Autodesk Inventor part; units mm, degrees
ref_plane "YZ Plane" through (0, 0, 0) normal (1, 0, 0) x (0, 1, 0)
ref_plane "XZ Plane" through (0, 0, 0) normal (0, 1, 0) x (-1, 0, 0)
ref_plane "XY Plane" through (0, 0, 0) normal (0, 0, 1) x (1, 0, 0)
sketch "Sketch1" plane through (0, 0, 0) normal (0, 0, 1) x (1, 0, 0)
  line L0 (2, 0) -> (65, 0)
  line L1 (65, 0) -> (65, 29)
  line L2 (65, 29) -> (2, 29)
  line L3 (0, 27) -> (0, 2)
  arc A0 (2, 29) -> (0, 27) centre (2, 27) ccw
  arc A1 (0, 2) -> (2, 0) centre (2, 2) ccw
  line L4 (20, 29) -> (20, 0)
  line L5 (55, 29) -> (55, 0)
  circle A2 centre (7, 24.5) radius 1.5
  circle A3 centre (7, 4.5) radius 1.5
  circle A4 centre (13.5, 24.5) radius 1.5
  circle A5 centre (13.5, 4.5) radius 1.5
  line L6 (65, 0) -> (65, -2.5)
  line L7 (65, -2.5) -> (55, -2.5)
  line L8 (55, -2.5) -> (55, 0)
  line L9 (55, 29) -> (55, 31.5)
  line L10 (55, 31.5) -> (65, 31.5)
  line L11 (65, 31.5) -> (65, 29)
  point P0 (0, 0)
  point P1 (0, 29)
  dimension "d0" = 65
  dimension "d1" = 29
  dimension "d2" = 2
  dimension "d3" = 20
  dimension "d4" = 10
  dimension "d5" = 3
  dimension "d6" = 3
  dimension "d7" = 4.5
  dimension "d8" = 4.5
  dimension "d9" = 20
  dimension "d10" = 3
  dimension "d11" = 3
  dimension "d12" = 20
  dimension "d13" = 6.5
  dimension "d14" = 7
  dimension "d24" = 2.5
  dimension "d25" = 2.5
extrude "Extrusion1" add sketch "Sketch1" along normal blind 5 contours L4 L2 L5 L0
extrude "Extrusion2" add sketch "Sketch1" along normal blind 7 contours A1 L3 A0 L2 L4 L0
extrude "Extrusion3" add sketch "Sketch1" along normal blind 26.25 contours L5 L2 L1 L0
sketch "Sketch2" plane through (55, 0, 5) normal (-1, 0, 0) x (0, 0, 1)
  line L0 (21.25, 29) -> (21.25, 0)
  circle A0 centre (21.25, 14.5) radius 10
  point P0 (-5, 0)
  point P1 (21.25, 4.5)
  point P2 (21.25, 24.5)
  dimension "d21" = 20
extrude "Extrusion4" cut sketch "Sketch2" against normal blind 20 contours L0 A0 picked at (15.0351, 13.318)
extrude "Extrusion5" add sketch "Sketch1" along normal blind 26.25 contours L0 L6 L7 L8 | L9 L10 L11 L2
sketch "Sketch4" plane through (55, 0, 5) normal (-1, 0, 0) x (0, 0, 1)
  circle A0 centre (13.75, 1.5095) radius 2.05
  circle A1 centre (13.75, 27.4905) radius 2.05
  line L0 (-5, -2.5) -> (21.25, -2.5)
  line L1 (-5, 31.5) -> (21.25, 31.5)
  line L2 (21.25, 31.5) -> (21.25, 24.5)
  point P0 (-5, 0)
  point P1 (8.125, -2.5)
  dimension "d28" = 4.1
  dimension "d29" = 4.1
  dimension "d30" = 25.981
  dimension "d31" = 4.0095
  dimension "d32" = 4.0095
  dimension "d33" = 7.5
extrude "Extrusion6" cut sketch "Sketch4" against normal blind 26.25
chamfer "Chamfer1" distance 2.5 angle 45 1 edges at (55, 0, 2.5)
chamfer "Chamfer2" distance 2.5 angle 45 1 edges at (55, 29, 2.5)
chamfer "Chamfer3" distance 6 angle 45 1 edges at (55, 14.5, 5)
chamfer "Chamfer4" distance 0.6 angle 45 6 edges at (20, 14.5, 7) (11, 0, 7) (0.5858, 0.5858, 7) (0, 14.5, 7) (0.5858, 28.4142, 7) (11, 29, 7)
equation "\"BendRadius\" = Thickness"
equation "\"BendReliefWidth\" = Thickness"
equation "\"BendReliefDepth\" = 0.5 * Thickness"
equation "\"CornerReliefSize\" = 4 * Thickness"
equation "\"MinimumRemnant\" = 2 * Thickness"
equation "\"TransitionRadius\" = BendRadius"
equation "\"JacobiRadiusSize\" = BendRadius"
equation "\"GapSize\" = Thickness"
properties part number "tool4_1"
The listing builds one solid part. Answer for the finished solid, in the listing's coordinates (mm). A direction names the side the tool comes from. Give positions to 0.01 mm unless a question says otherwise; leave off trailing zeros. Order: outer loops, then holes, each group sorted by start corner. A loop starts at its lowest first (then second) coordinate and runs counter-clockwise, first axis right, second up. Notation, with made-up numbers: (-36.75, 22) -> (-7.75, 22) arc R7 ccw to (-7.75, 26) -> close; hole circle Ø4 at (-17, 54.25). An arc over 180 degrees is marked (long way). Answer as a JSON object with one key per item and string values. Group by question number.
Item 1: A tool of negligible diameter and unlimited length cuts with its end or side. For faces 5 (the flat face through (10, 15, 7)), 6 (the cylindrical face through (12.39, 23.49, 3.45)), 7 (the flat face through (52, 14, 8)), from which of +Z, -Z, +X, -X, +Y, -Y can it reach the whole face along a straight path? Write none if from no direction.
Item 2: The part is cut by section B-B on z = 20. Write down the section's boundary in (x, y).
Item 3: Flat-ended cylindrical pins translate along their axes: pin 1 (6.5 mm diameter, centred on y = 1.51, z = 18.75, fed in from -X); pin 2 (5 mm diameter, centred on x = 13.5, y = 24.5, fed in from +Z); pin 3 (12 mm diameter, centred on x = 43.5, z = 5, fed in from -Y). Find the tip coordinate at first contact, or state that the pin passes through.
Item 4: The part is cut by section D-D on y = 14.5. Write down the section's boundary in (x, z), and give its area (3 significant figures).
Item 5: The part is cut by section A-A on x = 13.5. Write down the section's boundary in (y, z).
Item 6: Consider L1, parallel to Y at x = 7, z = 5.25; L2, parallel to X at y = 24, z = 3; L3, parallel to Y at x = 58.75, z = 18.75. Determine where each line is inside the solid, lowest interval first. Write a range as from..to.
Item 7: The part is cut by section C-C on z = 24.5. Write down the section's boundary in (x, y), and give its area (3 significant figures).
Item 8: Determine the mould class of faces 1 (the flat face through (34, 15, 5)), 2 (the flat face through (28, 29, 2)), 3 (the flat face through (53.7, 30.2, 5.4)), 4 (the flat face through (20, 15, 6)) for opening direction X: pulls with the +X half, pulls with the -X half, needs draft (parallel to the pull), parting line crosses it, or undercut.
Result set:
{
 "1": {"face 5": "+Z, -X, +Y, -Y", "face 6": "+Z, -Z", "face 7": "+Z, +Y, -Y"},
 "2": {"outline": "(55, -2.5) -> (65, -2.5) -> (65, -0.12) -> (55, -0.12) -> close; (55, 3.13) -> (65, 3.13) -> (65, 6.69) -> (55, 6.69) -> close; (55, 22.31) -> (65, 22.31) -> (65, 25.87) -> (55, 25.87) -> close; (55, 29.12) -> (65, 29.12) -> (65, 31.5) -> (55, 31.5) -> close"},
 "3": {"pin 1": "x = 55", "pin 2": "z = 7", "pin 3": "y = 0"},
 "4": {"outline": "(0, 0) -> (65, 0) -> (65, 16.25) -> (55, 16.25) -> (55, 11) -> (49, 5) -> (20, 5) -> (20, 6.4) -> (19.4, 7) -> (0.6, 7) -> (0, 6.4) -> close", "area": "495 mm²"},
 "5": {"outline": "(0, 0) -> (3, 0) -> (3, 7) -> (0.6, 7) -> (0, 6.4) -> close; (6, 0) -> (23, 0) -> (23, 7) -> (6, 7) -> close; (26, 0) -> (29, 0) -> (29, 6.4) -> (28.4, 7) -> (26, 7) -> close"},
 "6": {"L1": "0..3, 6..23, 26..29", "L2": "0..5.59, 8.41..12.09, 14.91..65", "L3": "-2.5..-0.54, 3.56..7.89, 21.11..25.44, 29.54..31.5"},
 "7": {"outline": "(55, -2.5) -> (65, -2.5) -> (65, 4.65) -> (55, 4.65) -> close; (55, 24.35) -> (65, 24.35) -> (65, 31.5) -> (55, 31.5) -> close", "area": "143 mm²"},
 "8": {"face 1": "undercut", "face 2": "needs draft", "face 3": "pulls with the -X half", "face 4": "undercut"}
}
